Job drawing, mm, ordinate dimensions from the low corner. One solid piece. Give positions to 0.01 mm unless a question says otherwise; leave off trailing zeros. Order: outer loops, then holes, each group sorted by start corner. A loop starts at its lowest first (then second) coordinate and runs counter-clockwise, first axis right, second up.
1. Slice it at C-C on x = 8. List the corners of the cut face in (y, z).
2. Slice it at A-A on z = 11.5. List the corners of the cut face in (x, y), and give its area (3 significant figures).
3. Slice it at B-B on y = 2.65. List the corners of the cut face in (x, z), and give its area (3 significant figures).
4. Drop a flat-ended pin along its axis: pin 1 Ø1.6 at (x, y) = (5.5, 3) entering from -Z. Give the stop position or say it passes through.
5. Probe line 1 (X direction, y = 1.2, z = 8.5); line 2 (Z direction, x = 124, y = 2.3); line 3 (Z direction, x = 8.5, y = 2.5). List the from-to ranges inside material, lowest first.
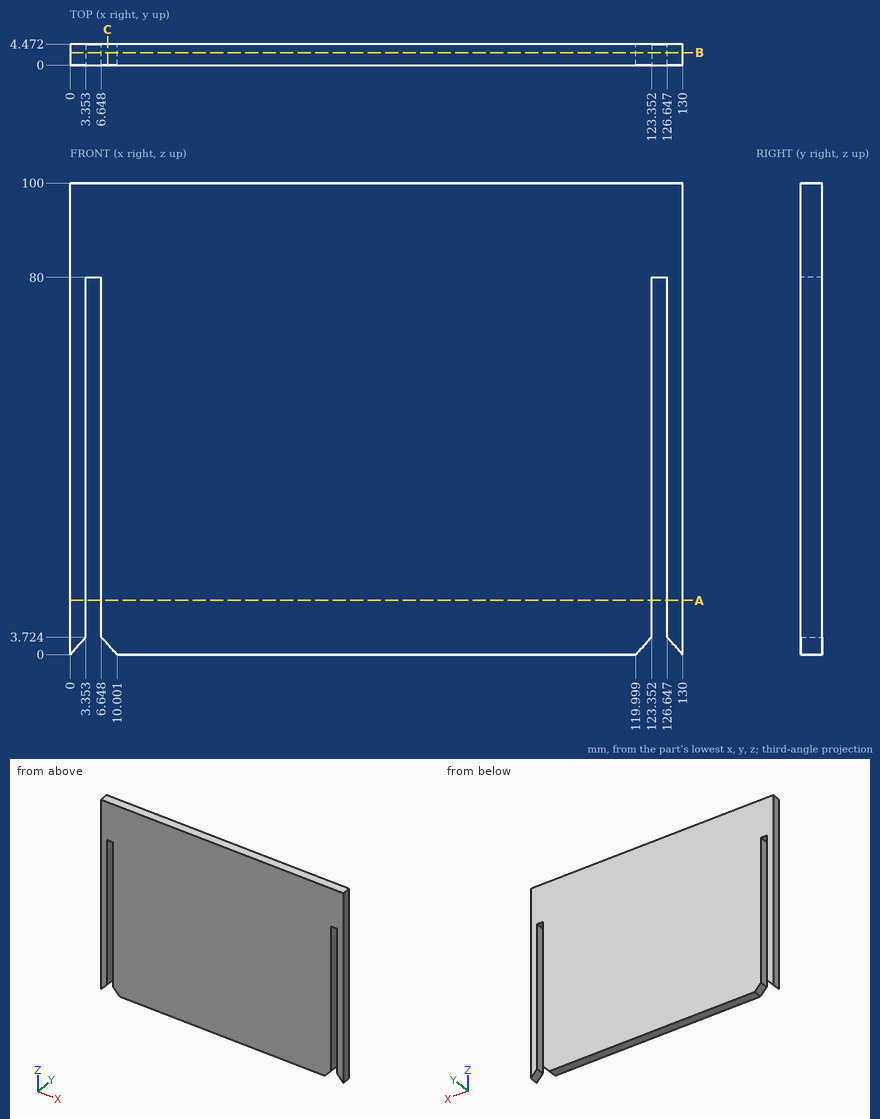
Data:
1. outline: (0, 2.22) - (4.47, 2.22) - (4.47, 100) - (0, 100) - close
2. outline: (0, 0) - (3.35, 0) - (3.35, 4.47) - (0, 4.47) - close; (6.65, 0) - (123.35, 0) - (123.35, 4.47) - (6.65, 4.47) - close; (126.65, 0) - (130, 0) - (130, 4.47) - (126.65, 4.47) - close
2. area: 552 mm2
3. outline: (0, 0) - (3.35, 3.72) - (3.35, 80) - (6.65, 80) - (6.65, 3.72) - (10, 0) - (120, 0) - (123.35, 3.72) - (123.35, 80) - (126.65, 80) - (126.65, 3.72) - (130, 0) - (130, 100) - (0, 100) - close
3. area: 12,400 mm2
4. pin 1: stops at z = 80
5. line 1: x = 0 to 3.35, 6.65 to 123.35, 126.65 to 130
5. line 2: z = 80 to 100
5. line 3: z = 1.67 to 100
